Design review of the part shown in the three views and the two pictorial views. Dimensions are in mm from the part's minimum x, y and z. Give positions to 0.01 mm unless a question says otherwise; leave off trailing zeros. Order: outer loops, then holes, each group sorted by start corner. A loop starts at its lowest first (then second) coordinate and runs counter-clockwise, first axis right, second up.
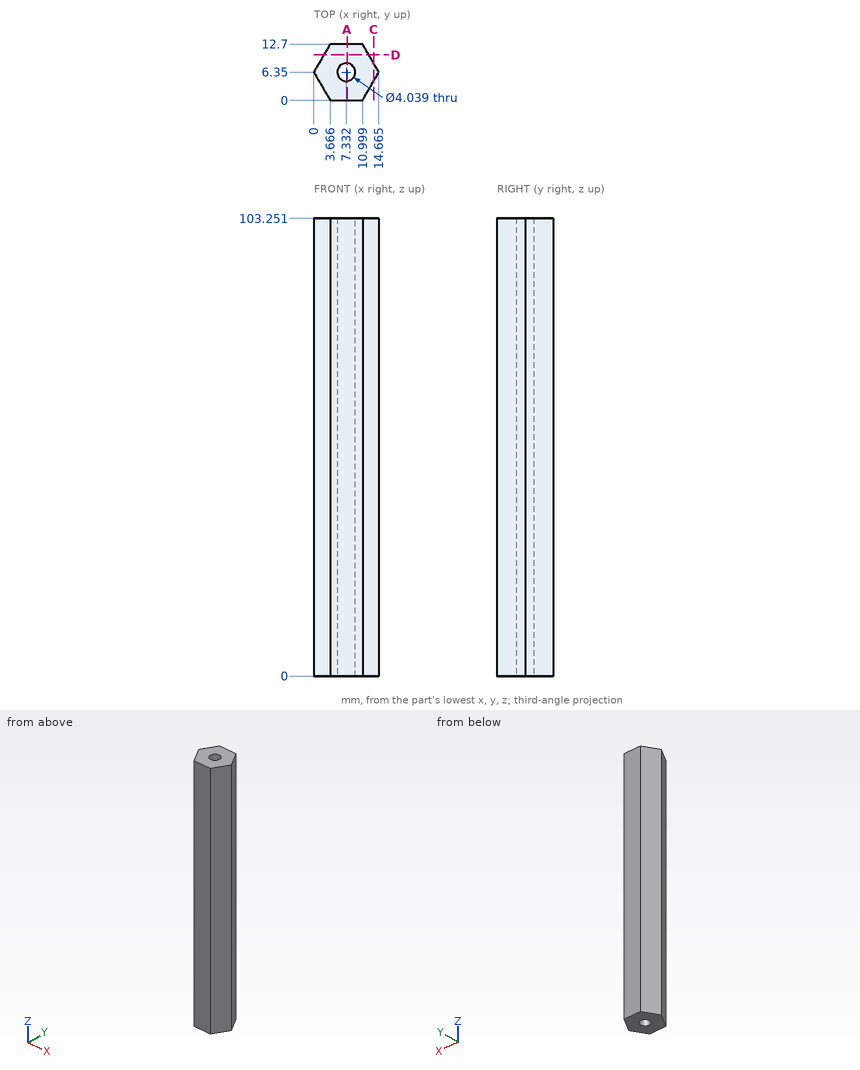
1) We need section C-C on x = 13.5. Give the boundary of the cut face in (y, z).
Answer sheet:
outline: (4.33, 0) - (8.37, 0) - (8.37, 103.25) - (4.33, 103.25) - close
2) We need section D-D on y = 10.25. Give the boundary of the cut face in (x, z), then the cut area to 3 significant figures.
Answer sheet:
outline: (2.25, 0) - (12.41, 0) - (12.41, 103.25) - (2.25, 103.25) - close
area: 1,050 mm2
3) We need section A-A on x = 7.5. Give the boundary of the cut face in (y, z).
Answer sheet:
outline: (0, 0) - (4.34, 0) - (4.34, 103.25) - (0, 103.25) - close; (8.36, 0) - (12.7, 0) - (12.7, 103.25) - (8.36, 103.25) - close
4) To check wall thickness, follow line 1 (X direction, y = 7.75, z = 63.5) (1 decimal); line 2 (Y direction, x = 7.75, z = 17.5) (1 decimal); line 3 (X direction, y = 6, z = 50) (1 decimal). State the ranges of each line that lie inside material, in increasing order.
Answer sheet:
line 1: x = 0.8 to 5.9, 8.8 to 13.9
line 2: y = 0 to 4.4, 8.3 to 12.7
line 3: x = 0.2 to 5.3, 9.3 to 14.5
5) Clearance check with flat-ended pins moving along their axes: pin 1 (2 mm diameter, centred on y = 4, z = 22.5, fed in from -X); pin 2 (5 mm diameter, centred on y = 6, z = 77.5, fed in from +X) (1 decimal). State where each tip first meets the part, or that it passes through.
Answer sheet:
pin 1: stops at x = 0.78
pin 2: stops at x = 14.7
